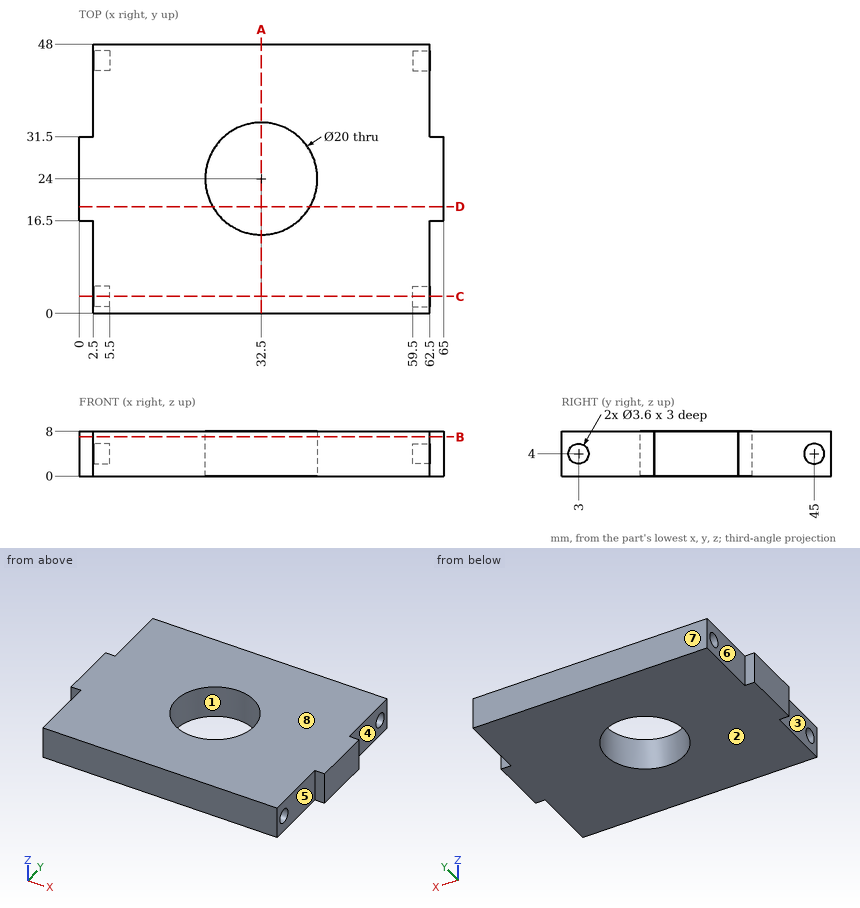
Could you check a few things on this drawing? It's one solid part, dimensions in mm from its lowest x, y, z. A direction names the side the tool comes from. Round coordinates to 2 decimals unless told otherwise and drop trailing zeros. Write each loop counter-clockwise with the first axis right and the second up, starting at its lowest first coordinate (ties: lowest second). Pieces come first, ordered by that corner, then holes. Notation, with made-up numbers: (1, -3) -> (29, -3) arc R15 cw to (29, 19) -> close; hole circle Ø8 at (70.5, 87). An arc over 180 degrees is marked (long way). One line per item, written item: value.
1) Suppose I cut it at A-A on x = 32.5. List the corners of the cut face in (y, z) for me, plus the area to 3 significant figures.
Filled sheet:
outline: (0, 0) -> (14, 0) -> (14, 8) -> (0, 8) -> close; (34, 0) -> (48, 0) -> (48, 8) -> (34, 8) -> close
area: 224 mm2
2) Suppose I cut it at D-D on y = 19. List the corners of the cut face in (x, z) for me.
Filled sheet:
outline: (0, 0) -> (23.84, 0) -> (23.84, 8) -> (0, 8) -> close; (41.16, 0) -> (65, 0) -> (65, 8) -> (41.16, 8) -> close
3) Suppose I cut it at C-C on y = 3. List the corners of the cut face in (x, z) for me, plus the area to 3 significant figures.
Filled sheet:
outline: (2.5, 0) -> (62.5, 0) -> (62.5, 2.2) -> (59.5, 2.2) -> (59.5, 5.8) -> (62.5, 5.8) -> (62.5, 8) -> (2.5, 8) -> (2.5, 5.8) -> (5.5, 5.8) -> (5.5, 2.2) -> (2.5, 2.2) -> close
area: 458 mm2
4) I'm going to push flat-ended pins straight in: pin 1 Ø0.8 at (x, z) = (64, 3) entering from +Y; pin 2 Ø1.8 at (y, z) = (45, 3.5) entering from -X; pin 3 Ø2 at (y, z) = (3, 4) entering from +X; pin 4 Ø1.5 at (y, z) = (25, 1.5) entering from -X. Where does each tip first touch, or does it pass through?
Filled sheet:
pin 1: stops at y = 31.5
pin 2: stops at x = 5.5
pin 3: stops at x = 59.5
pin 4: stops at x = 0
5) Suppose I cut it at B-B on z = 7. List the corners of the cut face in (x, y) for me, plus the area to 3 significant figures.
Filled sheet:
outline: (0, 16.5) -> (2.5, 16.5) -> (2.5, 0) -> (62.5, 0) -> (62.5, 16.5) -> (65, 16.5) -> (65, 31.5) -> (62.5, 31.5) -> (62.5, 48) -> (2.5, 48) -> (2.5, 31.5) -> (0, 31.5) -> close; hole circle Ø20 at (32.5, 24)
area: 2,640 mm2
6) If I drill on line 1 (Z direction, x = 3.45, y = 3); line 2 (Y direction, x = 61.85, z = 4); line 3 (X direction, y = 38.5, z = 7), over which ranges is the centre line in solid material (lowest first)? Write a range as [from, to].
Filled sheet:
line 1: z = [0, 2.2], [5.8, 8]
line 2: y = [0, 1.2], [4.8, 43.2], [46.8, 48]
line 3: x = [2.5, 62.5]
7) We'd pull the mould along X, two halves only. Please class the marked faces 1, 2 and 3: released by +X, released by -X, zero draft, split by the parting line, or undercut.
Filled sheet:
face 1: undercut
face 2: zero draft
face 3: released by -X
8) For the marked faces 4, 5, 6, 7 and 8, which set-ups out of +Z, -Z, +X, -X, +Y, -Y let a thin tool reach every point of the face, with its end or its side?
Filled sheet:
face 4: +Z, -Z, +X, +Y
face 5: +Z, -Z, +X, -Y
face 6: +Z, -Z, -X, +Y
face 7: +Z, -Z, +X, -X, +Y
face 8: +Z, +X, -X, +Y, -Y
